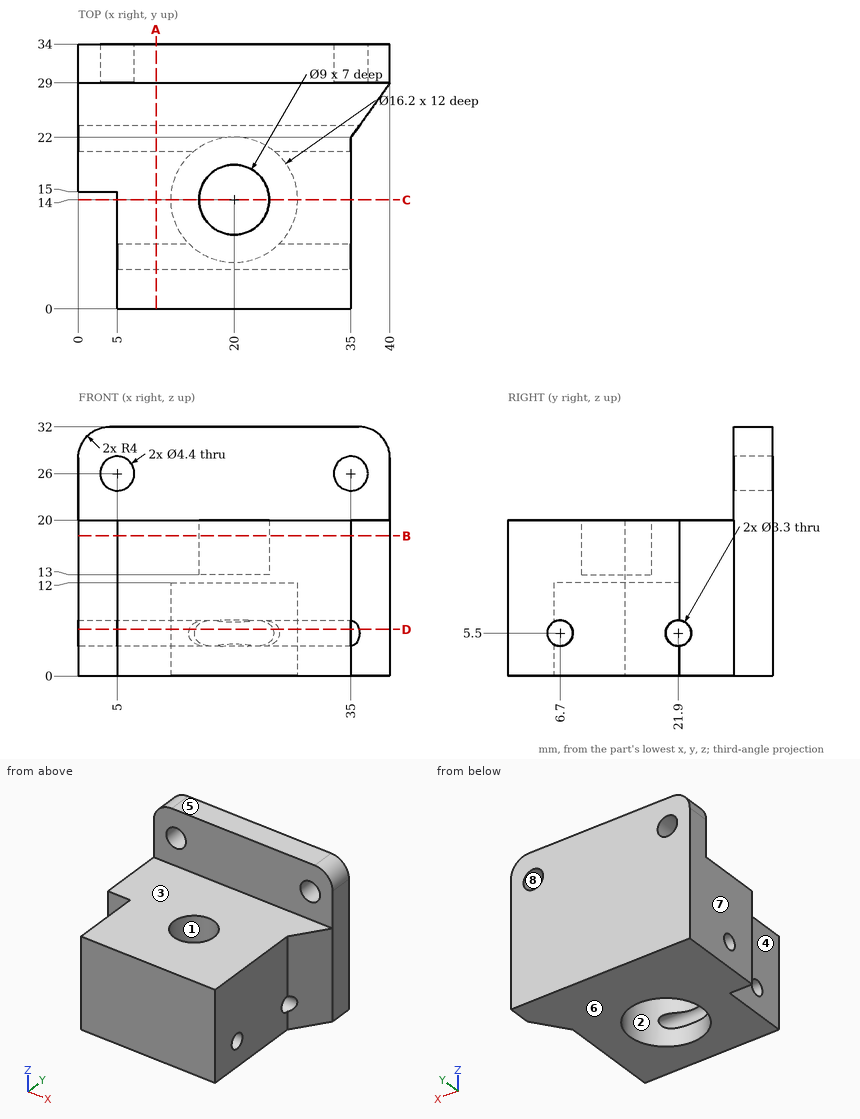
Input: dimensioned drawing with shaded views. Units: mm. Origin: part minimum x, y, z. A direction names the side the tool comes from. Give positions to 0.01 mm unless a question says otherwise; leave off trailing zeros. Write each loop counter-clockwise with the first axis right and the second up, starting at its lowest first coordinate (ties: lowest second). Pieces come first, ordered by that corner, then holes.
Q1. Section D-D, the plane z = 6. Output: boundary loops of the cut face in (x, y), plus the area to 3 significant figures.
Q2. Section B-B, the plane z = 18. Output: boundary loops of the cut face in (x, y), plus the area to 3 significant figures.
Q3. Material intervals for probe 1 along Z at (x, y) = (15, 6.7); probe 2 along Y at (x, z) = (20, 3.75); probe 3 along Y at (x, z) = (20, 15.75), sorted ascending.
Q4. First-contact query: P1, Ø4, axis at x = 35, z = 26, coming from the +Y side; P2, Ø10, axis at y = 6.5, z = 10, coming from the +X side; P3, Ø2, axis at x = 15.5, z = 25, coming from the -Y side; P4, Ø10, axis at x = 18.5, y = 14.5, coming from the +Z side. Flat tips, straight axial feed; report the tip coordinate or a pass-through.
Q5. Section C-C, the plane y = 14. Output: boundary loops of the cut face in (x, z).
Q6. Set-up query: the marked faces 1, 2, 3 and 4. Return all of +Z, -Z, +X, -X, +Y, -Y with unobstructed straight access to the full face (end or side cutting, diameter ignored); none if empty.
Q7. Pull-direction query (Z, two-part tool) for the marked faces 5, 6, 7 and 8; classes: pulls with the +Z half, pulls with the -Z half, needs draft (parallel to the pull), parting line crosses it, or undercut.
Q8. Section A-A, the plane x = 10. Output: boundary loops of the cut face in (y, z).
Filled in:
1. outline: (0, 15) - (5, 15) - (5, 8.27) - (14.27, 8.27) arc R8.1 cw to (14.94, 20.33) - (0, 20.33) - close; (0, 23.47) - (36.05, 23.47) - (40, 29) - (40, 34) - (0, 34) - close; (5, 0) - (35, 0) - (35, 5.13) - (5, 5.13) - close; (25.06, 20.33) arc R8.1 cw to (25.73, 8.27) - (35, 8.27) - (35, 20.33) - close
1. area: 777 mm2
2. outline: (0, 15) - (5, 15) - (5, 0) - (35, 0) - (35, 22) - (40, 29) - (40, 34) - (0, 34) - close; hole circle Ø9 at (20, 14)
2. area: 1,090 mm2
3. probe 1: z = 0 to 3.85, 7.15 to 20
3. probe 2: y = 0 to 5.9, 22.1 to 34
3. probe 3: y = 0 to 9.5, 18.5 to 34
4. P1: passes through
4. P2: stops at x = 35
4. P3: stops at y = 29
4. P4: stops at z = 20
5. outline: (5, 0) - (11.9, 0) - (11.9, 12) - (28.1, 12) - (28.1, 0) - (35, 0) - (35, 20) - (24.5, 20) - (24.5, 13) - (15.5, 13) - (15.5, 20) - (5, 20) - close
6. face 1: +Z
6. face 2: -Z
6. face 3: +Z, +X, -X, -Y
6. face 4: +Z, -Z, -X, -Y
7. face 5: pulls with the +Z half
7. face 6: pulls with the -Z half
7. face 7: needs draft
7. face 8: undercut
8. outline: (0, 0) - (34, 0) - (34, 32) - (29, 32) - (29, 20) - (0, 20) - close; hole circle Ø3.3 at (6.7, 5.5); hole circle Ø3.3 at (21.9, 5.5)
